from build123d import *

# Parameters (mm, degrees)
SKETCH1_R           = 42.55
BOSS_EXTRUDE1_DEPTH = 1
SKETCH2_R           = 42.55
SKETCH2_R_2         = 41.55
CUT_EXTRUDE1_DEPTH  = 102.547405362
SKETCH3_R           = 41.55
SKETCH3_R_2         = 41.05
CUT_EXTRUDE2_DEPTH  = 0.25


with BuildPart() as part:
    # Sketch1 → Boss-Extrude1 (new body)
    with BuildSketch(Plane(origin=(0, 0, 0), x_dir=(1, 0, 0), z_dir=(0, 1, 0))):
        with Locations(Location((-46.303063169, -6.602911423, 0), (0, 0, 270))):
            Circle(SKETCH1_R)
    extrude(amount=BOSS_EXTRUDE1_DEPTH)

    # Sketch2 → Cut-Extrude1 (cut, through all)
    with BuildSketch(Plane(origin=(0, 1, 0), x_dir=(1, 0, 0), z_dir=(0, 1, 0))):
        with Locations((-46.303063169, -6.602911423)):
            Circle(SKETCH2_R)
        with Locations(Location((-46.303063169, -6.602911423, 0), (0, 0, 270))):
            Circle(SKETCH2_R_2, mode=Mode.SUBTRACT)
    extrude(amount=-CUT_EXTRUDE1_DEPTH, mode=Mode.SUBTRACT)

    # Sketch3 → Cut-Extrude2 (cut)
    with BuildSketch(Plane(origin=(0, 1, 0), x_dir=(1, 0, 0), z_dir=(0, 1, 0))):
        with Locations(Location((-46.303063169, -6.602911423, 0), (0, 0, 270))):
            Circle(SKETCH3_R)
        with Locations(Location((-46.303063169, -6.602911423, 0), (0, 0, 270))):
            Circle(SKETCH3_R_2, mode=Mode.SUBTRACT)
    extrude(amount=-CUT_EXTRUDE2_DEPTH, mode=Mode.SUBTRACT)


solid = part.part
Could you check a few things on this model? Use its own coordinates, in mm. A direction names the side the tool comes from. Give positions to 0.01 mm unless a question says otherwise; leave off trailing zeros. Order: outer loops, then holes, each group sorted by start corner. A loop starts at its lowest first (then second) coordinate and runs counter-clockwise, first axis right, second up.
Item 1: If we section it at A-A, the plane x = -11.5: Write out the boundary of the cut face in (y, z), plus the area to 3 significant figures.
Item 2: For faces 3 (the face through (-6.1, 0.75, -2.8)), 4 (the face through (-46, 1, 6)), which set-ups out of +Z, -Z, +X, -X, +Y, -Y let a thin tool reach every point of the face, with its end or its side?
Item 3: If we section it at C-C, the plane y = 0.35: Write out the boundary of the cut face in (x, z).
Item 4: I need wall thicknesses on line 1 (X direction, y = 0.45, z = 19.5); line 2 (X direction, y = 0.65, z = 14.5); line 3 (Z direction, x = -61, y = 0.8). Which ranges of each line are inside material? Lowest first, please.
Item 5: If we mould it in two halves opening along Z, with no side actions, what happens to faces 1 (the face through (-18.2, 0.4, -24)), 2 (the face through (-46, 0, 6))? For each: pulls with the +Z half, pulls with the -Z half, needs draft (parallel to the pull), parting line crosses it, or undercut.
Item 6: If we section it at B-B, the plane z = -30: Write out the boundary of the cut face in (x, y).
Values:
1. outline: (0, -16.09) - (0.75, -16.09) - (0.75, -15.17) - (1, -15.17) - (1, 28.37) - (0.75, 28.37) - (0.75, 29.3) - (0, 29.3) - close
1. area: 44.9 mm2
2. face 3: +Y
2. face 4: +Z, -Z, +X, -X, +Y
3. outline: circle Ø83.1 at (-46.3, 6.6)
4. line 1: x = -85.8 to -6.81
4. line 2: x = -87.1 to -5.51
4. line 3: z = -31.73 to 44.93
5. face 1: parting line crosses it
5. face 2: needs draft
6. outline: (-65.97, 0) - (-26.64, 0) - (-26.64, 0.75) - (-27.72, 0.75) - (-27.72, 1) - (-64.89, 1) - (-64.89, 0.75) - (-65.97, 0.75) - close
